Check sheet for the modelled part. Datum: model origin and axes. Units: mm. Face numbers are marked on the shaded views. Round coordinates to 2 decimals unless told otherwise and drop trailing zeros. Write each loop counter-clockwise with the first axis right and the second up, starting at its lowest first coordinate (ties: lowest second). Pieces come first, ordered by that corner, then holes. Notation, with made-up numbers: M 17,-40 L 44,-40 A20 cw 44,-10 Z; hole C 7,49.5 d5. An arc over 180 degrees is marked long. Put each result on its own line as item: value.
```python
from build123d import *

# Parameters (mm, degrees)
IZIM1_W                              = 100
IZIM1_H                              = 50
IZIM1_R                              = 2.476303865
IZIM1_R_2                            = 9.5
IZIM1_R_3                            = 2.283039358
Y_KSEKLIK_EKSTR_ZYON1_DEPTH          = 8
M5_HELISARMAL_I_IN_Z_VANA_MATKAB_1_D = 5.2
KES_EKSTR_ZYON1_DEPTH                = 10
KES_EKSTR_ZYON1_DEPTH_BACK           = 10
IZIM4_R                              = 11.5
IZIM4_R_2                            = 1.25
M5_HELISARMAL_I_IN_Z_VANA_MATKAB_2_D = 5.2


with BuildPart() as part:
    # Çizim1 → Yükseklik-Ekstrüzyon1 (new body)
    # profile 1 of 6: a face of its own
    with BuildSketch(Plane.XY):
        with Locations((91.850220264, -26.688693098)):
            Rectangle(IZIM1_W, IZIM1_H)
        with Locations((131.850220264, -41.688693098)):
            Circle(IZIM1_R, mode=Mode.SUBTRACT)
        with Locations((111.850220264, -26.688693098)):
            Circle(IZIM1_R_2, mode=Mode.SUBTRACT)
        with Locations((131.850220264, -11.688693098)):
            Circle(IZIM1_R_3, mode=Mode.SUBTRACT)
    # profile 2 of 6: a face of its own
    with BuildSketch(Plane.XY):
        with Locations((-8.149779736, -26.688693098)):
            Rectangle(IZIM1_W, IZIM1_H)
        with Locations((-48.149779736, -41.688693098)):
            Circle(IZIM1_R, mode=Mode.SUBTRACT)
        with Locations((-28.149779736, -26.688693098)):
            Circle(IZIM1_R_2, mode=Mode.SUBTRACT)
        with Locations((-48.149779736, -11.688693098)):
            Circle(IZIM1_R_3, mode=Mode.SUBTRACT)
    # profile 3 of 6: a face of its own
    with BuildSketch(Plane.XY):
        with Locations((-48.149779736, -11.688693098)):
            Circle(IZIM1_R_3)
    # profile 4 of 6: a face of its own
    with BuildSketch(Plane.XY):
        with Locations((-48.149779736, -41.688693098)):
            Circle(IZIM1_R)
    # profile 5 of 6: a face of its own
    with BuildSketch(Plane.XY):
        with Locations((131.850220264, -11.688693098)):
            Circle(IZIM1_R_3)
    # profile 6 of 6: a face of its own
    with BuildSketch(Plane.XY):
        with Locations((131.850220264, -41.688693098)):
            Circle(IZIM1_R)
    extrude(amount=Y_KSEKLIK_EKSTR_ZYON1_DEPTH)

    # M5 Helisarmal için Zıvana matkabı1 (through all)
    with Locations(Plane.XY.offset(8)):
        with Locations((-48.149779736, -11.688693098), (-48.149779736, -41.688693098), (131.850220264, -41.688693098), (131.850220264, -11.688693098)):
            Hole(M5_HELISARMAL_I_IN_Z_VANA_MATKAB_1_D / 2)

    # Çizim4 → Kes-Ekstrüzyon1 (cut, two sides: drawn at the far end of the back side and taken through both)
    with BuildSketch(Plane(origin=(0, 0, 0), x_dir=(-1, 0, 0), z_dir=(0, 0, -1)).offset(-KES_EKSTR_ZYON1_DEPTH_BACK)):
        with Locations(Location((-41.850220264, -26.688693098, 0), (0, 0, 180))):
            Circle(IZIM4_R)
        with Locations(Location((-57.350220264, -11.188693098, 0), (0, 0, 180))):
            Circle(IZIM4_R_2)
        with Locations(Location((-56.781535146, -42.188693098, 0), (0, 0, 180))):
            Circle(IZIM4_R_2)
        with Locations(Location((-25.781535146, -41.329010258, 0), (0, 0, 180))):
            Circle(IZIM4_R_2)
        with Locations(Location((-26.350220264, -10.329010258, 0), (0, 0, 180))):
            Circle(IZIM4_R_2)
    extrude(amount=KES_EKSTR_ZYON1_DEPTH + KES_EKSTR_ZYON1_DEPTH_BACK, mode=Mode.SUBTRACT)

    # M5 Helisarmal için Zıvana matkabı2 (through all)
    with Locations(Plane(origin=(-18.149779736, -41.688693098, 8), x_dir=(1, 0, 0), z_dir=(0, 0, 1))):
        with Locations((0, 0), (120, 0)):
            Hole(M5_HELISARMAL_I_IN_Z_VANA_MATKAB_2_D / 2)


solid = part.part
```
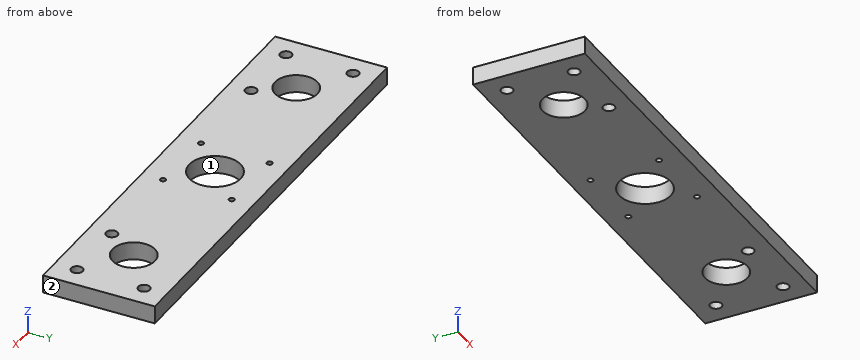
1. Scan lines: probe 1 along X at (y, z) = (-26.5, 5.25); probe 2 along X at (y, z) = (-18, 6.25); probe 3 along X at (y, z) = (-11, 3.5). Record each from-to range of solid material in increasing order.
Computed values:
probe 1: x = -58.15 to -37.65, -18.65 to 30.35, 53.35 to 102.35, 121.35 to 141.85
probe 2: x = -58.15 to -31.99, -24.31 to 34.32, 49.38 to 108.01, 115.69 to 141.85
probe 3: x = -58.15 to -50.66, -45.64 to 25.3, 27.4 to 56.11, 58.59 to 129.34, 134.36 to 141.85
2. Cross-section at A-A (x = -29). Enter the section's corners in (y, z).
Computed values:
outline: M -51.69,0 L -36.15,0 L -36.15,8 L -51.69,8 Z; M -17.23,0 L -1.69,0 L -1.69,8 L -17.23,8 Z
3. Depth check by flat-ended pin: pin 1 Ø2 at (x, y) = (26.35, -10.33) entering from +Z. Enter the tip coordinate at first touch or a pass-through.
Computed values:
pin 1: passes through
4. Cross-section at C-C (z = 4.5). Count the separate pieces of the cut face and the enclosed holes in it, then the cut area to 3 significant figures.
Computed values:
separate pieces: 1
enclosed holes: 13
area: 8,870 mm2
5. Cross-section at D-D (x = 113). Enter the section's corners in (y, z), then the cut area to 3 significant figures.
Computed values:
outline: M -51.69,0 L -36.12,0 L -36.12,8 L -51.69,8 Z; M -17.26,0 L -1.69,0 L -1.69,8 L -17.26,8 Z
area: 249 mm2
6. Release check for a two-part mould opening along Y. For the marked faces 1 and 2 record: +Y half, -Y half, draft (parallel to the pull), parting line (faces both ways), or undercut.
Computed values:
face 1: undercut
face 2: draft
7. Cross-section at B-B (y = -32). Enter the section's corners in (x, z), then the cut area to 3 significant figures.
Computed values:
outline: M -58.15,0 L -36.03,0 L -36.03,8 L -58.15,8 Z; M -20.27,0 L 31.65,0 L 31.65,8 L -20.27,8 Z; M 52.05,0 L 103.97,0 L 103.97,8 L 52.05,8 Z; M 119.73,0 L 141.85,0 L 141.85,8 L 119.73,8 Z
area: 1,180 mm2
